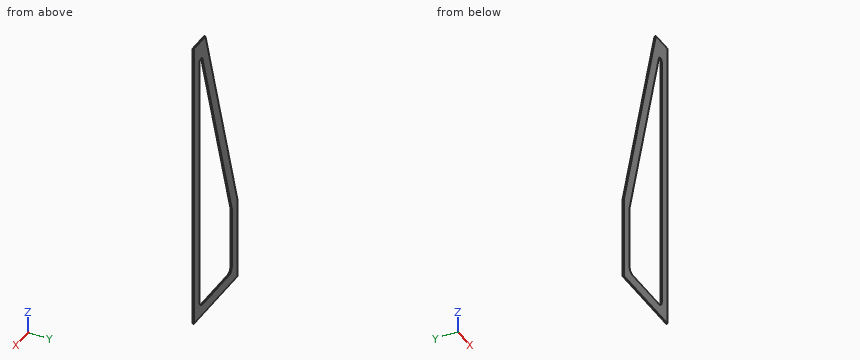
from build123d import *

# Parameters (mm, degrees)
BOSS_EXTRUDE1_DEPTH = 6.35


with BuildPart() as part:
    # Sketch1 → Boss-Extrude1 (new body)
    with BuildSketch(Plane(origin=(0, 0, 0), x_dir=(1, 0, 0), z_dir=(0, 1, 0))):
        Polygon((0, 0), (0, -1384.3), (-101.6, -1384.3), (-381, -381), (-381, 0), align=None)
        with BuildLine():
            Line((-329.268912254, -377.402099424), (-75.377865092, -1289.10176878))
            ThreePointArc((-75.377865092, -1289.10176878), (-61.858495332, -1297.3737261), (-50.8, -1286.019946218))
            Line((-50.8, -1286.019946218), (-50.8, -76.2))
            ThreePointArc((-50.8, -76.2), (-58.239487758, -58.239487758), (-76.2, -50.8))
            Line((-76.2, -50.8), (-304.8, -50.8))
            ThreePointArc((-304.8, -50.8), (-322.760512242, -58.239487758), (-330.2, -76.2))
            Line((-330.2, -76.2), (-330.2, -370.58797196))
            ThreePointArc((-330.2, -370.58797196), (-329.966151586, -374.026694742), (-329.268912254, -377.402099424))
        make_face(mode=Mode.SUBTRACT)
    extrude(amount=BOSS_EXTRUDE1_DEPTH)


solid = part.part
Work out the finished part from the listing and answer in its coordinate system (mm). Round coordinates to 2 decimals unless told otherwise and drop trailing zeros. Order: outer loops, then holes, each group sorted by start corner. A loop starts at its lowest first (then second) coordinate and runs counter-clockwise, first axis right, second up. Notation, with made-up numbers: M 3.5,-9.5 L 24.5,-9.5 A33 ccw 24.5,20.5 Z; hole C -29.75,29.5 d3. An arc over 180 degrees is marked long. Put each result on its own line as item: value. Start each with the question number.
Q1. Section C-C, the plane x = -277 is taken. Write down the section's boundary in (y, z), and give its area (3 significant figures).
Q2. Section A-A, the plane z = 92.5 is taken. Write down the section's boundary in (x, y).
Q3. Straight lines are drawn through the part: L1, parallel to X at y = 0.5, z = 332; L2, parallel to X at y = 2, z = 695. For each, find the intervals that lie inside material, in ascending order. Write a range as [from, to].
Q4. Section B-B, the plane y = 3.75 is taken. Write down the section's boundary in (x, z), and give its area (3 significant figures).
Findings below:
1. outline: M 0,0 L 6.35,0 L 6.35,50.8 L 0,50.8 Z; M 0,565.1 L 6.35,565.1 L 6.35,754.45 L 0,754.45 Z
1. area: 1,530 mm^2
2. outline: M -381,0 L -330.2,0 L -330.2,6.35 L -381,6.35 Z; M -50.8,0 L 0,0 L 0,6.35 L -50.8,6.35 Z
3. L1: x = [-381, -330.2], [-50.8, 0]
3. L2: x = [-293.56, -240.82], [-50.8, 0]
4. outline: M -381,0 L 0,0 L 0,1384.3 L -101.6,1384.3 L -381,381 Z; hole M -330.2,76.2 A25.4 ccw -304.8,50.8 L -76.2,50.8 A25.4 ccw -50.8,76.2 L -50.8,1286.02 A12.7 ccw -75.38,1289.1 L -329.27,377.4 A25.4 ccw -330.2,370.59 Z
4. area: 158,000 mm^2
